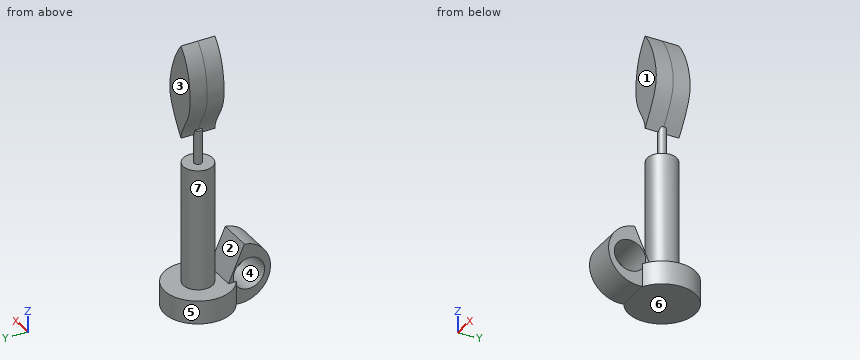
```python
from build123d import *

# Parameters (mm, degrees)
F0_R      = 25.0862676095
F0_R_2    = 9.9212052261
F1_DEPTH  = 17.526
F2_R      = 11.0191356669
F3_DEPTH  = 108.712
F5_R      = 2.8727507543
F6_DEPTH  = 25.4
F8_DEPTH  = 12.7
F9_R      = 11.7410453839
F10_DEPTH = 12.7
F12_DEPTH = 12.7


with BuildPart() as f1:
    # F0 (on Top) → F1 (new body)
    with BuildSketch(Plane.XY):
        Circle(F0_R)
        Circle(F0_R_2, mode=Mode.SUBTRACT)
    extrude(amount=F1_DEPTH)

    # F2 (on Top) → F3 (join)
    with BuildSketch(Plane.XY):
        Circle(F2_R)
    extrude(amount=F3_DEPTH)

    # F5 (on offset) → F6 (join)
    with BuildSketch(Plane.XY.offset(134.112)):
        Circle(F5_R)
    extrude(amount=-F6_DEPTH)

    # F7 (on Right) → F8 (join, symmetric)
    with BuildSketch(Plane.YZ):
        with BuildLine():
            Line((-14.0056908131, 13.5905332863), (-27.6115936243, 44.3398724095))
            ThreePointArc((-27.6115936243, 44.3398724095), (-47.0539529538, 19.3601672357), (-22.0104921012, 0))
            Line((-22.0104921012, 0), (-14.0056908131, 13.5905332863))
        make_face()
    extrude(amount=F8_DEPTH, both=True)

    # F9 (on Right) → F10 (cut, symmetric)
    with BuildSketch(Plane.YZ):
        with Locations((-31.1411302537, 21.0428796709)):
            Circle(F9_R)
    extrude(amount=F10_DEPTH, both=True, mode=Mode.SUBTRACT)

    # F11 (on Front) → F12 (join, symmetric)
    with BuildSketch(Plane.XZ):
        with BuildLine():
            add(Edge.make_bspline(
                [(0, 201.5375494957), (8.2067918749, 191.5956386678), (17.6385011209, 165.7506647475), (14.33397457, 150.9642153978), (0, 130.8100919055)],
                knots=[0, 0, 0, 0, 0.4810826992, 1, 1, 1, 1], degree=3))
            add(Edge.make_bspline(
                [(0, 201.5375494957), (-9.1203246266, 192.0092403889), (-13.1277565836, 171.0788275856), (-11.6600287617, 151.1036541195), (0, 137.038230896), (0, 130.8100919055)],
                knots=[0, 0, 0, 0, 0.3852312794, 0.6845969407, 1, 1, 1, 1], degree=3))
        make_face()
    extrude(amount=F12_DEPTH, both=True)


solid = f1.part
```
Check sheet for the modelled part. Datum: model origin and axes. Units: mm. Face numbers are marked on the shaded views. A direction names the side the tool comes from. Give positions to 0.01 mm unless a question says otherwise; leave off trailing zeros. Order: outer loops, then holes, each group sorted by start corner. A loop starts at its lowest first (then second) coordinate and runs counter-clockwise, first axis right, second up. Notation, with made-up numbers: (-31, 80) -> (-8, 80) arc R35 ccw to (-8, 118) -> close; hole circle Ø1 at (57, 1). An arc over 180 degrees is marked (long way). Return JSON: item names as keys, results as strings.
1. Cross-section at B-B, the plane z = 98.5. Record the cut outline in (x, y), plus the area to 3 significant figures.
From the geometry:
{"outline": "circle Ø22.04 at (0, 0)", "area": "381 mm^2"}
2. Set-up check for the marked faces 5, 6 and 7: record each of +Z, -Z, +X, -X, +Y, -Y from which the full face is reachable in a straight line by a thin tool's end or side.
From the geometry:
{"face 5": "+Z, -Z", "face 6": "-Z, +X, -X, +Y", "face 7": "none"}
3. Mould release check, pull along Y, two halves, no side actions. Record for the marked faces 1, 2, 3 and 4: +Y half, -Y half, draft (parallel to the pull), parting line (faces both ways), or undercut.
From the geometry:
{"face 1": "-Y half", "face 2": "undercut", "face 3": "+Y half", "face 4": "undercut"}
4. Cross-section at D-D, the plane x = -17.5. Record the cut outline in (y, z), plus the area to 3 significant figures.
From the geometry:
{"outline": "(-17.97, 0) -> (17.97, 0) -> (17.97, 17.53) -> (-17.97, 17.53) -> close", "area": "630 mm^2"}
5. Cross-section at A-A, the plane x = -8. Count the separate pieces of the cut face and the enclosed holes in it, plus the area to 3 significant figures.
From the geometry:
{"separate pieces": "2", "enclosed holes": "1", "area": "3,700 mm^2"}
6. Material ranges on probe 1 along Z at (x, y) = (19.5, -6); probe 2 along Z at (x, y) = (-8, -23.5); probe 3 along Z at (x, y) = (-4, 6), recorded low to high. Write a range as [from, to].
From the geometry:
{"probe 1": "[0, 17.53]", "probe 2": "[-0.14, 12.13], [29.96, 35.05]", "probe 3": "[0, 108.71], [141.81, 196.63]"}
7. Go/stop test with flat-tipped pins: P1, Ø1.9, axis at y = -20.5, z = 16.5, coming from the +X side; P2, Ø2, axis at x = 14.5, z = 162, coming from the -Y side; P3, Ø14, axis at x = -3.5, y = -9, coming from the +Z side; P4, Ø8, axis at x = -0.5, z = 168.5, coming from the +Y side. Record where each tip stops, or that it passes through.
From the geometry:
{"P1": "x = 15.72", "P2": "y = -12.7", "P3": "z = 201.54", "P4": "y = 12.7"}
